CAD build for the part. Positions are in the model's coordinates, mm. A direction names the side the tool comes from. Coordinates: 2 decimals unless noted, no trailing zeros. Loops run counter-clockwise (first coordinate to the right, second up) from the corner with the lowest first, then second, coordinate; pieces in that order, holes last. Notation, with made-up numbers: (24.5, 2) -> (81.5, 2) arc R20 cw to (81.5, 12) -> close; hole circle Ø8 at (77.25, 11.5). An arc over 180 degrees is marked (long way). Write each question's results on one line, items separated by ' | '.
from build123d import *

# Parameters (mm, degrees)
SKETCH5_R               = 41
CUT_EXTRUDE2_DEPTH      = 200
SKETCH10_R              = 99
SKETCH10_R_2            = 42
CUT_EXTRUDE3_DEPTH      = 1
CUT_EXTRUDE3_DEPTH_BACK = 2.1


with BuildPart() as part:
    # Sketch3 → Revolve1 (revolve)
    with BuildSketch(Plane(origin=(0, 0, 0), x_dir=(0, 0, -1), z_dir=(1, 0, 0))):
        Polygon((0, 0), (100, 0), (50, 200), (0, 200), align=None)
    revolve(axis=Axis((0, 0, 0), (0, 1, 0)))

    # Sketch5 → Cut-Extrude2 (cut)
    with BuildSketch(Plane(origin=(0, 0, 0), x_dir=(1, 0, 0), z_dir=(0, 1, 0))):
        Circle(SKETCH5_R)
    extrude(amount=CUT_EXTRUDE2_DEPTH, mode=Mode.SUBTRACT)

    # Sketch7 → Cut-Revolve1 (revolve, cut)
    with BuildSketch(Plane(origin=(0, 0, 0), x_dir=(0, 0, -1), z_dir=(1, 0, 0))):
        Polygon((96.923058984, 2), (48.048058984, 197.5), (42.5, 197.5), (42.5, 2), align=None)
    revolve(axis=Axis((0, 0, 0), (0, -1, 0)), mode=Mode.SUBTRACT)

    # Sketch10 → Cut-Extrude3 (cut, two sides)
    with BuildSketch(Plane.XZ) as cut_extrude3_sk:
        Circle(SKETCH10_R)
        Circle(SKETCH10_R_2, mode=Mode.SUBTRACT)
    extrude(amount=CUT_EXTRUDE3_DEPTH, mode=Mode.SUBTRACT)
    extrude(cut_extrude3_sk.sketch, amount=-CUT_EXTRUDE3_DEPTH_BACK, mode=Mode.SUBTRACT)


solid = part.part
1) Slice it at A-A (x = 0). Write the cut outline in (y, z).
Outcome:
outline: (0, -100) -> (200, -50) -> (200, -41) -> (0, -41) -> (0, -42) -> (2.1, -42) -> (2.1, -42.5) -> (197.5, -42.5) -> (197.5, -48.05) -> (2.1, -96.9) -> (2.1, -99) -> (0, -99) -> close; (0, 41) -> (200, 41) -> (200, 50) -> (0, 100) -> (0, 99) -> (2.1, 99) -> (2.1, 96.9) -> (197.5, 48.05) -> (197.5, 42.5) -> (2.1, 42.5) -> (2.1, 42) -> (0, 42) -> close
2) Two-plate mould, pull along X, no slides. Class faces 1 (the flat face through (73, 2.1, -66)), 2 (the conical face through (67.45, 123.62, 14.98)), 3 (the flat face through (-41, 200, 4)): pulls with the +X half, pulls with the -X half, needs draft (parallel to the pull), parting line crosses it, or undercut.
Outcome:
face 1: undercut | face 2: parting line crosses it | face 3: needs draft
3) Slice it at C-C (y = 101). Write the cut outline in (x, z), then the cut area to 3 significant figures.
Outcome:
outline: circle Ø149.5 at (0, 0); circle Ø85 at (0, 0); hole circle Ø144.35 at (0, 0); hole circle Ø82 at (0, 0) | area: 1,580 mm^2
4) Slice it at D-D (y = 70). Write the cut outline in (x, z).
Outcome:
outline: circle Ø165 at (0, 0); circle Ø85 at (0, 0); hole circle Ø159.85 at (0, 0); hole circle Ø82 at (0, 0)
5) Which spindle directions (+Z, -Z, +X, -X, +Y, -Y) get a long thin tool onto all of the face, cutting with end or side? Do faces 4 (the flat face through (40.2, 0, 9.1)), 5 (the cylindrical face through (-12.888, 1.035, 98.158)). Say none if no direction does.
Outcome:
face 4: +Z, -Z, +X, -X, -Y | face 5: -Y
6) Slice it at B-B (z = 0). Write the cut outline in (x, y), then the cut area to 3 significant figures.
Outcome:
outline: (-100, 0) -> (-99, 0) -> (-99, 2.1) -> (-96.9, 2.1) -> (-48.05, 197.5) -> (-42.5, 197.5) -> (-42.5, 2.1) -> (-42, 2.1) -> (-42, 0) -> (-41, 0) -> (-41, 200) -> (-50, 200) -> close; (41, 0) -> (42, 0) -> (42, 2.1) -> (42.5, 2.1) -> (42.5, 197.5) -> (48.05, 197.5) -> (96.9, 2.1) -> (99, 2.1) -> (99, 0) -> (100, 0) -> (50, 200) -> (41, 200) -> close | area: 1,650 mm^2
7) Drill centre lines: L1, parallel to X at y = 21.5, z = -17; L2, parallel to Z at x = 0, y = 1.7 (3 decimals); L3, parallel to X at y = 61, z = 0. Where is each one in solid material? Low to high. Write a range as from..to.
Outcome:
L1: x = -93.09..-90.46, -38.95..-37.31, 37.31..38.95, 90.46..93.09 | L2: z = -99.575..-99, -42..-41, 41..42, 99..99.575 | L3: x = -84.75..-82.17, -42.5..-41, 41..42.5, 82.17..84.75
8) Pin check, flat tips, straight feed: pin 1 (1 mm diameter, centred on x = -37.5, z = -14, fed in from -Y); pin 2 (1.5 mm diameter, centred on x = -68.5, y = 36.5, fed in from +Z); pin 3 (10 mm diameter, centred on x = 15.5, y = 153.5, fed in from -Z); pin 4 (1.5 mm diameter, centred on x = 32.5, y = 122.5, fed in from +Z). Stop position of each tip, or through.
Outcome:
pin 1: passes through | pin 2: stops at z = 60.61 | pin 3: stops at z = -61.37 | pin 4: stops at z = 61.74
